Source: CAD feature listing. Evaluate the final solid. Frame: model axes, mm. A direction names the side the tool comes from. Give positions to 0.01 mm unless a question says otherwise; leave off trailing zeros. Loops run counter-clockwise (first coordinate to the right, second up) from the corner with the lowest first, then second, coordinate; pieces in that order, holes last. Notation, with made-up numbers: M 73.25,57 L 84.25,57 A38 ccw 84.25,96 Z; hole C 25,74 d11. An arc over 180 degrees is marked long. Write item = value, one per line.
from build123d import *

# Parameters (mm, degrees)
CYLINDER040_R               = 5.5
CYLINDER040_DEPTH           = 8
CYLINDER039_R               = 12
CYLINDER039_DEPTH           = 2
CYLINDER038_R               = 7.85
CYLINDER038_DEPTH           = 8
CHAMFER003068012002091_SIZE = 0.4


with BuildPart() as cylinder040:
    # Cylinder040 → Cylinder040 (new body)
    with BuildSketch(Plane.XY.offset(-2)):
        Circle(CYLINDER040_R)
    extrude(amount=CYLINDER040_DEPTH)


with BuildPart() as cylinder039:
    # Cylinder039 → Cylinder039 (new body)
    with BuildSketch(Plane.XY.offset(4)):
        Circle(CYLINDER039_R)
    extrude(amount=CYLINDER039_DEPTH)


with BuildPart() as bearing_remover_bottom:
    # Cylinder038 → Cylinder038 (new body)
    with BuildSketch(Plane.XY.offset(-2)):
        Circle(CYLINDER038_R)
    extrude(amount=CYLINDER038_DEPTH)

    # Fusion001002012036: union Cylinder039
    add(cylinder039.part)

    # Cut001042: cut Cylinder040
    add(cylinder040.part, mode=Mode.SUBTRACT)

    # Chamfer003068012002091
    chamfer003068012002091_edges = [bearing_remover_bottom.edges().sort_by_distance(p)[0] for p in [
        (-12, 0, 6),
        (-12, 0, 4),
        (-7.85, 0, -2),
        (-5.5, 0, 6),
        (-5.5, 0, -2),
    ]]
    chamfer(chamfer003068012002091_edges, length=CHAMFER003068012002091_SIZE)


with BuildPart() as bearing_remover_bottom_1:
    # Chamfer003068012002091 placement: moved
    add(bearing_remover_bottom.part.moved(Location((0, 0, 6))))


solid = bearing_remover_bottom_1.part
1. Material intervals for probe 1 along Y at (x, z) = (0, 7.25); probe 2 along Y at (x, z) = (-2.5, 4.75); probe 3 along Z at (x, y) = (-5.25, 10), sorted ascending. Write a range as from..to.
Derived:
probe_1 = -7.85..-5.5, 5.5..7.85
probe_2 = -7.44..-4.9, 4.9..7.44
probe_3 = 10..12
2. Cut plane C-C, the plane z = 4.75. Return the cut outline in (x, y).
Derived:
outline = C 0,0 d15.7; hole C 0,0 d11
3. Pull-direction query (X, two-part tool) for faces 1 (the cylindrical face through (-1.19, -5.37, 7.95)), 2 (the flat face through (-2, 6, 4)), 3 (the cylindrical face through (-11.99, 0.53, 10.99)); classes: +X half, -X half, draft (parallel to the pull), parting line (faces both ways), or undercut.
Derived:
face_1 = undercut
face_2 = draft
face_3 = parting line
4. Cut plane A-A, the plane y = 0. Return the cut outline in (x, z), then the cut area to 3 significant figures.
Derived:
outline = M -12,10.4 L -11.6,10 L -7.85,10 L -7.85,4.4 L -7.45,4 L -5.9,4 L -5.5,4.4 L -5.5,11.6 L -5.9,12 L -11.6,12 L -12,11.6 Z; M 5.5,4.4 L 5.9,4 L 7.45,4 L 7.85,4.4 L 7.85,10 L 11.6,10 L 12,10.4 L 12,11.6 L 11.6,12 L 5.9,12 L 5.5,11.6 Z
area = 53.4 mm²
5. First-contact query: pin 1 Ø6 at (x, y) = (-6.5, -6) entering from -Z; pin 2 Ø2 at (y, z) = (4, 10.5) entering from -X; pin 3 Ø4 at (y, z) = (-7, 5.5) entering from +X. Flat tips, straight axial feed; report the tip coordinate or a pass-through.
Derived:
pin_1 = 4
pin_2 = -11.62
pin_3 = 6.05
6. Reachability of faces 4 (the cylindrical face through (-5.786, 5.305, 7.161)), 5 (the flat face through (5, -5, 12)) from +Z, -Z, +X, -X, +Y, -Y: full face, straight path, thin tool, end or side. Return the list, or none.
Derived:
face_4 = -Z
face_5 = +Z, +X, -X, +Y, -Y
